Autodesk Inventor part; units mm, degrees
ref_plane "YZ Plane" through (0, 0, 0) normal (1, 0, 0) x (0, 1, 0)
ref_plane "XZ Plane" through (0, 0, 0) normal (0, 1, 0) x (-1, 0, 0)
ref_plane "XY Plane" through (0, 0, 0) normal (0, 0, 1) x (1, 0, 0)
sketch "Sketch1" plane through (0, 0, 0) normal (0, 0, 1) x (1, 0, 0)
  circle A0 centre (0, 0) radius 12.7
  dimension "d0" = 25.4
extrude "Extrusion1" add sketch "Sketch1" along normal blind 56.896
sketch "Sketch2" plane through (0, 0, 56.896) normal (0, 0, 1) x (1, 0, 0)
  circle A0 centre (0, 0) radius 6.35
  dimension "d4" = 12.7
hole "Hole1" at (0, 0, 56.896) direction (0, 0, -1) diameter 12.7 end through all
sketch "Sketch5" plane through (0, 0, 56.896) normal (0, 0, 1) x (1, 0, 0)
  circle A0 centre (0, 0) radius 33.5915
  dimension "d12" = 67.183
extrude "Extrusion2" add sketch "Sketch5" along normal blind 9.525
sketch "Sketch6" plane through (0, 0, 66.421) normal (0, 0, 1) x (1, 0, 0)
  circle A0 centre (0, 0) radius 6.35
hole "Hole2" at (0, 0, 66.421) direction (0, 0, -1) diameter 12.7 end through all
properties part number "SubSprocketNoTeeth"
The model under review builds one solid part; all positions refer to its coordinate system, in mm. Give positions to 0.01 mm unless a question says otherwise; leave off trailing zeros. Write each loop counter-clockwise with the first axis right and the second up, starting at its lowest first coordinate (ties: lowest second). Pieces come first, ordered by that corner, then holes. Notation, with made-up numbers: M 34.25,25 L 63.25,25 A29 ccw 63.25,57 Z; hole C -5.5,48 d11. An arc over 180 degrees is marked long. Write item = value, one per line. Start each with the question number.
Q1. We need section C-C (z = 23.5). State the section outline as (x, y) points, plus the area to 3 significant figures.
Q2. For line 1 (Y direction, x = 0, z = 53.5); line 2 (Z direction, x = -2.5, y = 18); line 3 (X direction, y = -20, z = 62), list the stretches that pass through material, from the lowest coordinate up.
Q3. Clearance check with flat-ended pins moving along their axes: pin 1 (1 mm diameter, centred on y = -2.5, z = 55.5, fed in from +X); pin 2 (20 mm diameter, centred on x = 6, y = 15.5, fed in from -Z); pin 3 (4 mm diameter, centred on x = -8.5, y = 19.5, fed in from -Z); pin 4 (12 mm diameter, centred on y = -5.5, z = 40.5, fed in from -X). State where each tip first meets the part, or that it passes through.
Q4. We need section D-D (z = 62). State the section outline as (x, y) points.
Q5. Mouldability with a two-part tool opening along Y and no side actions: class faces 1 (the face through (14, 0, 56.896)), 2 (the face through (-2.75, 12.4, 28.05)), 3 (the face through (6.2, 1.38, 32.75)) as released by +Y, released by -Y, zero draft, split by the parting line, or undercut.
Q6. We need section A-A (x = 0). State the section outline as (y, z) points.
Result set:
q1.outline = C 0,0 d25.4; hole C 0,0 d12.7
q1.area = 380 mm2
q2.line_1 = -12.7 to -6.35, 6.35 to 12.7
q2.line_2 = 56.9 to 66.42
q2.line_3 = -26.99 to 26.99
q3.pin_1 = 12.54
q3.pin_2 = 0
q3.pin_3 = 56.9
q3.pin_4 = -12.7
q4.outline = C 0,0 d67.18; hole C 0,0 d12.7
q5.face_1 = zero draft
q5.face_2 = split by the parting line
q5.face_3 = undercut
q6.outline = M -33.59,56.9 L -12.7,56.9 L -12.7,0 L -6.35,0 L -6.35,66.42 L -33.59,66.42 Z; M 6.35,0 L 12.7,0 L 12.7,56.9 L 33.59,56.9 L 33.59,66.42 L 6.35,66.42 Z
